from build123d import *

# Parameters (mm, degrees)
SKETCH_1_RX         = 15
SKETCH_1_RY         = 8
EXTRUDE_1_DEPTH     = 2
SKETCH_2_W          = 35
SKETCH_2_H          = 15
CUT_EXTRUDE_1_DEPTH = 141.815482103


with BuildPart() as part:
    # 草图1 → 凸台-拉伸1 (new body)
    with BuildSketch(Plane(origin=(0, 0, 0), x_dir=(1, 0, 0), z_dir=(0, 1, 0))):
        Polygon((-107.5, 38), (-10, 38), (-10, 40), (10, 40), (10, 38), (107.5, 38), (107.5, 40), (122.5, 40), (122.5, 38), (135, 38), (135, -38), (122.5, -38), (122.5, -40), (107.5, -40), (107.5, -38), (10, -38), (10, -40), (-10, -40), (-10, -38), (-107.5, -38), (-107.5, -40), (-122.5, -40), (-122.5, -38), (-135, -38), (-135, 38), (-122.5, 38), (-122.5, 40), (-107.5, 40), align=None)
        with Locations(Location((-65, 0), (0, 0, 90))):
            Ellipse(SKETCH_1_RX, SKETCH_1_RY, mode=Mode.SUBTRACT)
        with Locations(Location((65, 0), (0, 0, 90))):
            Ellipse(SKETCH_1_RX, SKETCH_1_RY, mode=Mode.SUBTRACT)
    extrude(amount=EXTRUDE_1_DEPTH)

    # 草图2 → 切除-拉伸1 (cut, through all)
    with BuildSketch(Plane.XZ):
        with Locations((-112.5, 24.5)):
            Rectangle(SKETCH_2_W, SKETCH_2_H)
    cut_extrude_1 = extrude(amount=-CUT_EXTRUDE_1_DEPTH, mode=Mode.SUBTRACT)

    # 镜向1: 切除-拉伸1 across plane
    add(cut_extrude_1.mirror(Plane(origin=(0, 0, 0), x_dir=(0, 0, 1), z_dir=(1, 0, 0))), mode=Mode.SUBTRACT)


solid = part.part
Work out the finished part from the listing and answer in its coordinate system (mm). Give positions to 0.01 mm unless a question says otherwise; leave off trailing zeros. Order: outer loops, then holes, each group sorted by start corner. A loop starts at its lowest first (then second) coordinate and runs counter-clockwise, first axis right, second up. Notation, with made-up numbers: (-15, 86) -> (-10, 86) arc R26 ccw to (-10, 119) -> close; hole circle Ø9 at (-29.75, 85). An arc over 180 degrees is marked (long way). Answer as a JSON object with one key per item and string values. Group by question number.
1. Section D-D on x = -33 is taken. Determine the outline of the cut face in (y, z), plus the area to 3 significant figures.
2. Section A-A on x = 112.5 is taken. Determine the outline of the cut face in (y, z), plus the area to 3 significant figures.
3. A flat-ended cylindrical pin translates along its axis: pin 1 Ø1 at (x, y) = (-84, 1) entering from -Z. Find the tip coordinate at first contact, or state that the pin passes through.
4. Consider line 1 along X through (y, z) = (0.35, 31.5); line 2 along X through (y, z) = (1.35, -1); line 3 along Z through (x, y) = (12.5, 1.85). Determine where each line is inside the solid, lowest interval first. Write a range as [from, to].
5. Section B-B on y = 0.5 is taken. Count the separate pieces of the cut face and the enclosed holes in it, plus the area to 3 significant figures.
Result sheet:
{
 "1": {"outline": "(0, -38) -> (2, -38) -> (2, 38) -> (0, 38) -> close", "area": "152 mm^2"},
 "2": {"outline": "(0, -40) -> (2, -40) -> (2, 17) -> (0, 17) -> close; (0, 32) -> (2, 32) -> (2, 40) -> (0, 40) -> close", "area": "130 mm^2"},
 "3": {"pin 1": "stops at z = -38"},
 "4": {"line 1": "x = [-135, -130], [-95, 95], [130, 135]", "line 2": "x = [-135, -72.98], [-57.02, 57.02], [72.98, 135]", "line 3": "z = [-38, 38]"},
 "5": {"separate pieces": "1", "enclosed holes": "4", "area": "18,900 mm^2"}
}
